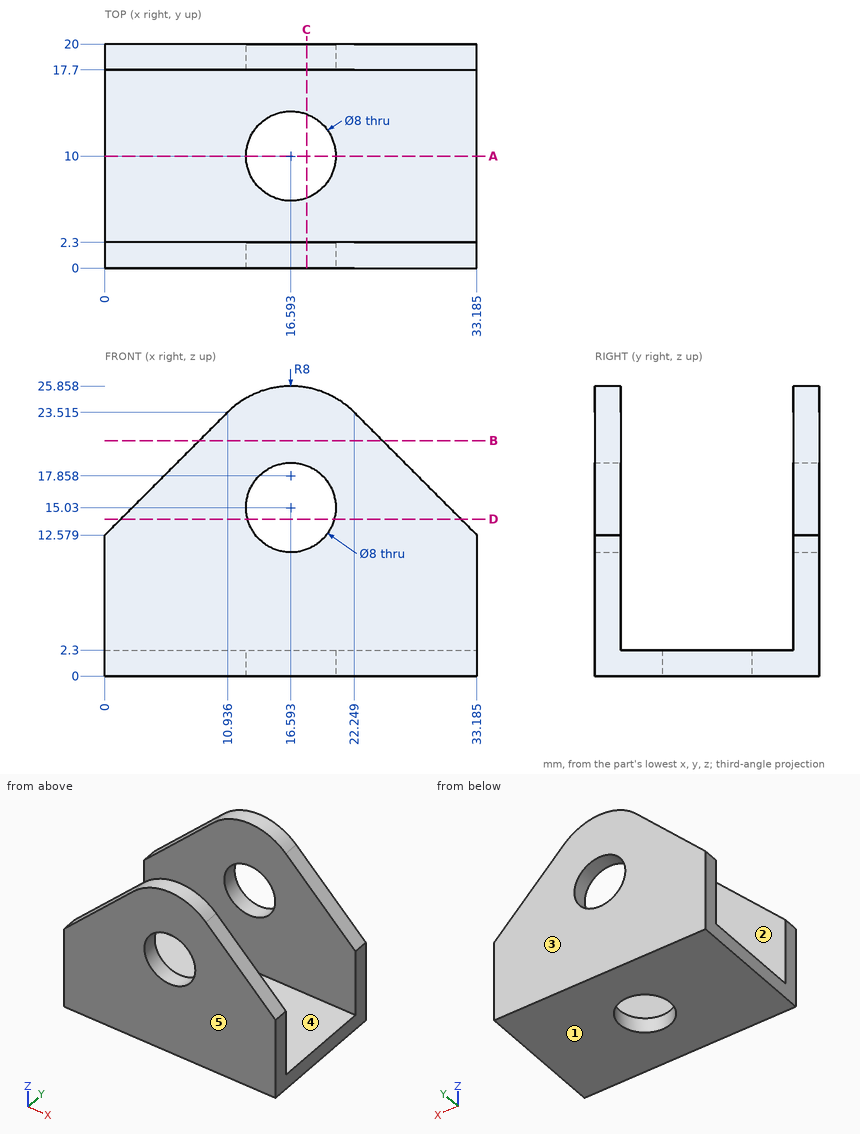
The figure shows three views and two pictorial views of one solid part (mm, origin at its lowest corner). Answer the questions. A direction names the side the tool comes from. Give positions to 0.01 mm unless a question says otherwise; leave off trailing zeros. Write each loop counter-clockwise with the first axis right and the second up, starting at its lowest first coordinate (ties: lowest second). Pieces come first, ordered by that corner, then holes. Notation, with made-up numbers: (47.5, -15) -> (71.5, -15) arc R25 ccw to (71.5, 4) -> close; hole circle Ø2 at (65, 88). An arc over 180 degrees is marked (long way). Use one line per item in the form item = value.
1) Straight lines are drawn through the part: probe 1 along Y at (x, z) = (11, 18.75); probe 2 along Z at (x, y) = (3, 14.25); probe 3 along Z at (x, y) = (18.5, 19.25) (1 decimal). For each, find the intervals that lie inside material, in ascending order.
Result:
probe_1 = 0 to 2.3, 17.7 to 20
probe_2 = 0 to 2.3
probe_3 = 0 to 11.5, 18.5 to 25.6
2) For a pull along Y with two mould halves and no side action, classify the marked faces 1, 2 and 3 as +Y half, -Y half, draft (parallel to the pull), parting line (faces both ways), or undercut.
Result:
face_1 = draft
face_2 = undercut
face_3 = +Y half
3) Section A-A on y = 10 is taken. Write down the section's boundary in (x, z) (1 decimal).
Result:
outline = (0, 0) -> (12.6, 0) -> (12.6, 2.3) -> (0, 2.3) -> close; (20.6, 0) -> (33.2, 0) -> (33.2, 2.3) -> (20.6, 2.3) -> close
4) Section C-C on x = 18 is taken. Write down the section's boundary in (y, z) (1 decimal).
Result:
outline = (0, 0) -> (6.3, 0) -> (6.3, 2.3) -> (2.3, 2.3) -> (2.3, 11.3) -> (0, 11.3) -> close; (0, 18.8) -> (2.3, 18.8) -> (2.3, 25.7) -> (0, 25.7) -> close; (13.7, 0) -> (20, 0) -> (20, 11.3) -> (17.7, 11.3) -> (17.7, 2.3) -> (13.7, 2.3) -> close; (17.7, 18.8) -> (20, 18.8) -> (20, 25.7) -> (17.7, 25.7) -> close
5) A tool of negligible diameter and unlimited length cuts with its end or side. For the marked faces 4 and 5, from which of +Z, -Z, +X, -X, +Y, -Y can it reach the whole face along a straight path? Write none if from no direction.
Result:
face_4 = +Z, +X, -X
face_5 = +Z, -Z, +X, -X, -Y
6) Each of these flat-tipped pins is pushed along its axis until it touches: P1, Ø7, axis at x = 16.59, z = 15.03, coming from the -Y side; P2, Ø7.5, axis at x = 12.5, y = 13, coming from the +Z side. Where does it stop, or does it pass through?
Result:
P1 = through
P2 = 2.3
7) Section D-D on z = 14 is taken. Write down the section's boundary in (x, y) (1 decimal), plus the area to 3 significant figures.
Result:
outline = (1.4, 0) -> (12.7, 0) -> (12.7, 2.3) -> (1.4, 2.3) -> close; (1.4, 17.7) -> (12.7, 17.7) -> (12.7, 20) -> (1.4, 20) -> close; (20.5, 0) -> (31.8, 0) -> (31.8, 2.3) -> (20.5, 2.3) -> close; (20.5, 17.7) -> (31.8, 17.7) -> (31.8, 20) -> (20.5, 20) -> close
area = 104 mm²
8) Section B-B on z = 21 is taken. Write down the section's boundary in (x, y) (1 decimal).
Result:
outline = (8.4, 0) -> (24.8, 0) -> (24.8, 2.3) -> (8.4, 2.3) -> close; (8.4, 17.7) -> (24.8, 17.7) -> (24.8, 20) -> (8.4, 20) -> close
